Autodesk Inventor part; units mm, degrees
ref_plane "YZ Plane" through (0, 0, 0) normal (1, 0, 0) x (0, 1, 0)
ref_plane "XZ Plane" through (0, 0, 0) normal (0, 1, 0) x (-1, 0, 0)
ref_plane "XY Plane" through (0, 0, 0) normal (0, 0, 1) x (1, 0, 0)
sketch "Sketch1" plane through (0, 0, 0) normal (1, 0, 0) x (0, 1, 0)
  line L0 (-12.7, 12.7) -> (12.7, 12.7)
  line L1 (12.7, 12.7) -> (12.7, -12.7)
  line L2 (12.7, -12.7) -> (-12.7, -12.7)
  line L3 (-12.7, -12.7) -> (-12.7, 12.7)
  line L4 (-11.1125, 11.1125) -> (11.1125, 11.1125)
  line L5 (11.1125, 11.1125) -> (11.1125, -10.8514)
  line L6 (11.1125, -10.8514) -> (-11.1125, -10.8514)
  line L7 (-11.1125, -10.8514) -> (-11.1125, 11.1125)
  point P0 (0, 0)
  point P1 (0, 12.7)
  point P2 (-12.7, 0)
  dimension "d0" = 25.4
  dimension "d1" = 25.4
  dimension "d2" = 1.5875
  dimension "d3" = 1.5875
  dimension "d4" = 1.5875
extrude "Extrusion1" add sketch "Sketch1" along normal blind 711.2
sketch "Sketch2" plane through (0, -12.7, 12.7) normal (0, 0, 1) x (1, 0, 0)
  circle A0 centre (9.525, 12.7) radius 6.35
  circle A1 centre (701.675, 12.7) radius 6.35
  line L0 (711.2, 25.4) -> (711.2, 0)
  line L1 (0, 0) -> (0, 25.4)
  line L2 (0, 0) -> (711.2, 0)
  circle A2 centre (355.6, 12.7) radius 6.35
  point P0 (0, 12.7)
  point P1 (395.7549, 0)
  point P2 (355.6, 0)
  dimension "d7" = 12.7
  dimension "d8" = 9.525
  dimension "d9" = 12.7
  dimension "d10" = 9.525
  dimension "d17" = 12.7
  dimension "d23" = 355.6
  dimension "BarLengthRef" = 711.2
extrude "Extrusion2" cut sketch "Sketch2" against normal blind 50.8 contours A0 | A1
extrude "Extrusion4" cut sketch "Sketch2" against normal blind 25.4 contours A2
fillet "Fillet1" radius 6.35 1 edges at (711.2, 12.7, 0)
fillet "Fillet2" radius 6.35 1 edges at (711.2, -12.7, 0)
equation "\"d1\" = d0"
equation "\"d3\" = d2"
equation "\"d4\" = d2"
equation "\"d9\" = d7"
equation "\"d10\" = d8"
equation "\"d17\" = d7"
equation "\"d23\" = 0.5 * BarLengthRef"
equation "\"XLS_Barlength\" = 711.2"
properties part number "2018 Long Bar Offset center"
Build history of the part. All positions in model axes, mm. A direction names the side the tool comes from. Give positions to 0.01 mm unless a question says otherwise; leave off trailing zeros. Write each loop counter-clockwise with the first axis right and the second up, starting at its lowest first coordinate (ties: lowest second). Pieces come first, ordered by that corner, then holes. Notation, with made-up numbers: (64, -2) - (77, -2) arc R12 ccw to (77, 20) - close; hole circle Ø6 at (44.25, 43). An arc over 180 degrees is marked (long way). Use one line per item in the form item = value. Start each with the question number.
1. Band-saw the part on B-B on z = -5. Write the cut outline in (x, y), plus the area to 3 significant figures.
2. Drop flat-ended pins along their axis: pin 1 Ø8 at (y, z) = (-5, 8) entering from -X; pin 2 Ø10 at (x, y) = (701.675, 0) entering from -Z. Give the stop position or say it passes through.
3. Band-saw the part on A-A on x = 355.6. Write the cut outline in (y, z).
4. Two-plate mould, pull along Y, no slides. Class faces 3 (the face through (351, 6, -12.7)), 4 (the face through (347, -12.7, 0)), 5 (the face through (15.58, 1.91, -11.76)): released by +Y, released by -Y, zero draft, split by the parting line, or undercut.
5. 3-axis set-ups, long thin cutter, end or side, ignore diameter. For faces 1 (the face through (351, 5, -10.851)), 2 (the face through (695.33, 0.28, 11.92)): which of +Z, -Z, +X, -X, +Y, -Y reach the whole face in a straight line?
6. Probe line 1 (Z direction, x = 359.5, y = 8); line 2 (Y direction, x = 55.5, z = -6); line 3 (Y direction, x = 355.6, z = 11.65). List the from-to ranges inside material, lowest first. Write a range as [from, to].
7. Band-saw the part on C-C on x = 596.5. Write the cut outline in (y, z).
Conclusion:
q1.outline = (0, -12.7) - (704.85, -12.7) arc R6.35 ccw to (709.05, -11.11) - (0, -11.11) - close; (0, 11.11) - (709.05, 11.11) arc R6.35 ccw to (704.85, 12.7) - (0, 12.7) - close
q1.area = 2,250 mm²
q2.pin_1 = 0
q2.pin_2 = through
q3.outline = (-12.7, -12.7) - (-6.35, -12.7) - (-6.35, -10.85) - (-11.11, -10.85) - (-11.11, 11.11) - (-6.35, 11.11) - (-6.35, 12.7) - (-12.7, 12.7) - close; (6.35, -12.7) - (12.7, -12.7) - (12.7, 12.7) - (6.35, 12.7) - (6.35, 11.11) - (11.11, 11.11) - (11.11, -10.85) - (6.35, -10.85) - close
q4.face_3 = zero draft
q4.face_4 = released by -Y
q4.face_5 = undercut
q5.face_1 = +X, -X
q5.face_2 = +Z, -Z
q6.line_1 = [-12.7, -10.85], [11.11, 12.7]
q6.line_2 = [-12.7, -11.11], [11.11, 12.7]
q6.line_3 = [-12.7, -6.35], [6.35, 12.7]
q7.outline = (-12.7, -12.7) - (12.7, -12.7) - (12.7, 12.7) - (-12.7, 12.7) - close; hole (-11.11, -10.85) - (11.11, -10.85) - (11.11, 11.11) - (-11.11, 11.11) - close
